```python
from build123d import *

# Parameters (mm, degrees)
SKETCH1_W           = 180
SKETCH1_H           = 77
SKETCH1_R           = 1.5
SKETCH1_R_2         = 1.500742376
BOSS_EXTRUDE1_DEPTH = 3
FILLET1_R           = 3
CUT_EXTRUDE1_DEPTH  = 3
SKETCH3_R           = 1.5
CUT_EXTRUDE2_DEPTH  = 3
SKETCH4_R           = 1.5
CUT_EXTRUDE3_DEPTH  = 3
SKETCH5_W           = 20
SKETCH5_H           = 34
BOSS_EXTRUDE2_DEPTH = 20
SKETCH6_R           = 1.5
CUT_EXTRUDE4_DEPTH  = 3


with BuildPart() as part:
    # Sketch1 → Boss-Extrude1 (new body)
    with BuildSketch(Plane(origin=(0, 0, 0), x_dir=(1, 0, 0), z_dir=(0, 1, 0))):
        Rectangle(SKETCH1_W, SKETCH1_H)
        with Locations(Location((-87, 35.25, 0), (0, 0, 270))):
            Circle(SKETCH1_R, mode=Mode.SUBTRACT)
        with Locations(Location((-87, -35.25, 0), (0, 0, 90))):
            Circle(SKETCH1_R, mode=Mode.SUBTRACT)
        with Locations(Location((-35.005408935, 34.5, 0), (0, 0, 270))):
            Circle(SKETCH1_R, mode=Mode.SUBTRACT)
        with Locations(Location((-35.005408935, -34.5, 0), (0, 0, 90))):
            Circle(SKETCH1_R, mode=Mode.SUBTRACT)
        with Locations(Location((74.494591065, 33.15, 0), (0, 0, 270))):
            Circle(SKETCH1_R_2, mode=Mode.SUBTRACT)
        with Locations(Location((74.494591065, -33.15, 0), (0, 0, 270))):
            Circle(SKETCH1_R, mode=Mode.SUBTRACT)
    extrude(amount=BOSS_EXTRUDE1_DEPTH)

    # Fillet1
    fillet1_edges = [part.edges().sort_by_distance(p)[0] for p in [
        (90, 1.5, 38.5),
        (-90, 1.5, 38.5),
        (-90, 1.5, -38.5),
        (90, 1.5, -38.5),
    ]]
    fillet(fillet1_edges, radius=FILLET1_R)

    # Sketch2 → Cut-Extrude1 (cut)
    with BuildSketch(Plane(origin=(0, 3, 0), x_dir=(1, 0, 0), z_dir=(0, 1, 0))):
        with BuildLine():
            Line((-62, 14.5), (-42, 14.5))
            ThreePointArc((-42, 14.5), (-41.292893219, 14.792893219), (-41, 15.5))
            Line((-41, 15.5), (-41, 28.5))
            ThreePointArc((-41, 28.5), (-41.292893219, 29.207106781), (-42, 29.5))
            Line((-42, 29.5), (-62, 29.5))
            ThreePointArc((-62, 29.5), (-62.707106781, 29.207106781), (-63, 28.5))
            Line((-63, 28.5), (-63, 15.5))
            ThreePointArc((-63, 15.5), (-62.707106781, 14.792893219), (-62, 14.5))
        make_face()
    extrude(amount=-CUT_EXTRUDE1_DEPTH, mode=Mode.SUBTRACT)

    # Sketch3 → Cut-Extrude2 (cut)
    with BuildSketch(Plane(origin=(0, 3, 0), x_dir=(1, 0, 0), z_dir=(0, 1, 0))):
        with Locations(Location((-79.5, 3.75, 0), (0, 0, 270))):
            Circle(SKETCH3_R)
        with Locations(Location((-42.5, 3.75, 0), (0, 0, 270))):
            Circle(SKETCH3_R)
        with Locations(Location((-42.5, -33.25, 0), (0, 0, 270))):
            Circle(SKETCH3_R)
        with Locations(Location((-79.5, -33.25, 0), (0, 0, 270))):
            Circle(SKETCH3_R)
    extrude(amount=-CUT_EXTRUDE2_DEPTH, mode=Mode.SUBTRACT)

    # Sketch4 → Cut-Extrude3 (cut)
    with BuildSketch(Plane(origin=(0, 3, 0), x_dir=(1, 0, 0), z_dir=(0, 1, 0))):
        with Locations(Location((-30.005408935, 24.25, 0), (0, 0, 270))):
            Circle(SKETCH4_R)
        with Locations(Location((52.994591065, 24.25, 0), (0, 0, 270))):
            Circle(SKETCH4_R)
        with Locations(Location((51.994591065, -24.25, 0), (0, 0, 270))):
            Circle(SKETCH4_R)
        with Locations(Location((-23.005408935, -24.25, 0), (0, 0, 270))):
            Circle(SKETCH4_R)
    extrude(amount=-CUT_EXTRUDE3_DEPTH, mode=Mode.SUBTRACT)

    # Sketch5 → Boss-Extrude2 (add)
    with BuildSketch(Plane.XZ):
        with Locations((40, 1.5)):
            Rectangle(SKETCH5_W, SKETCH5_H)
    extrude(amount=BOSS_EXTRUDE2_DEPTH)

    # Sketch6 → Cut-Extrude4 (cut)
    with BuildSketch(Plane.XZ):
        with Locations(Location((-14.5, -35.25, 0), (0, 0, 270))):
            Circle(SKETCH6_R)
        with Locations(Location((4.5, -35.25, 0), (0, 0, 270))):
            Circle(SKETCH6_R)
        with Locations(Location((4.5, 35.25, 0), (0, 0, 270))):
            Circle(SKETCH6_R)
        with Locations(Location((-14.5, 35.25, 0), (0, 0, 270))):
            Circle(SKETCH6_R)
        with Locations(Location((-5, -30.25, 0), (0, 0, 270))):
            Circle(SKETCH6_R)
        with Locations(Location((-5, 30.25, 0), (0, 0, 270))):
            Circle(SKETCH6_R)
    extrude(amount=-CUT_EXTRUDE4_DEPTH, mode=Mode.SUBTRACT)


solid = part.part
```
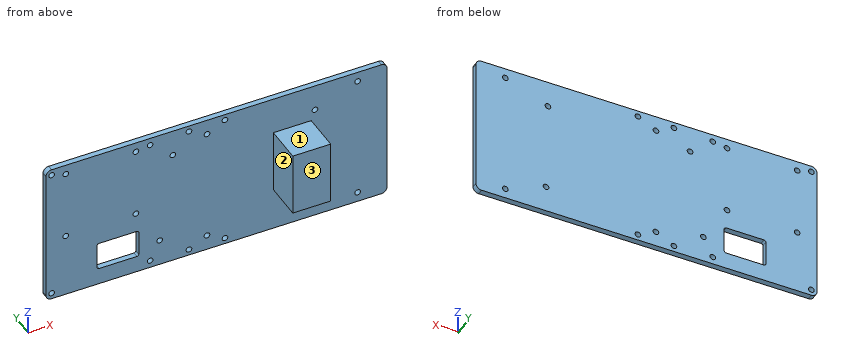
Geometry: final body of the model. Coordinates: model frame, mm. Face numbers are marked on the shaded views. A direction names the side the tool comes from. Give positions to 0.01 mm unless a question says otherwise; leave off trailing zeros. Loops run counter-clockwise (first coordinate to the right, second up) from the corner with the lowest first, then second, coordinate; pieces in that order, holes last. Notation, with made-up numbers: (37, -6) -> (45, -6) arc R7 cw to (45, -1) -> close; hole circle Ø3 at (11.5, -19). An arc over 180 degrees is marked (long way). Use CSV: the item, a comma, the result in double quotes.
(1) First-contact query: P1, Ø3, axis at x = 1, z = -5.5, coming from the -Y side. Flat tip, straight axial feed; report the tip coordinate or a pass-through.
From the geometry:
P1,"y = 0"
(2) Cut plane C-C (x = -66). Output: boundary loops of the cut face in (y, z), plus the area to 3 significant figures.
From the geometry:
outline,"(0, -38.5) -> (3, -38.5) -> (3, 38.5) -> (0, 38.5) -> close"
area,"231 mm^2"
(3) Access query for the marked faces 1, 2 and 3. Directions: +Z, -Z, +X, -X, +Y, -Y. A direction counts if a zero-diameter tool reaches every point of the face in a straight line with its end or side. Return the directions, or none.
From the geometry:
face 1,"+Z, +X, -X, -Y"
face 2,"+Z, -Z, -X, -Y"
face 3,"+Z, -Z, +X, -X, -Y"
(4) Ray query, line 1 along X through (y, z) = (2.4, -3.75); line 2 along X through (y, z) = (2, -24.25); line 3 along Z through (x, y) = (-87, 1). Return the intervals inside material, ascending. Write a range as [from, to].
From the geometry:
line 1,"[-90, -81], [-78, -44], [-41, 90]"
line 2,"[-90, -63], [-41, -31.51], [-28.51, 51.49], [54.49, 90]"
line 3,"[-38.5, -36.75], [-33.75, 33.75], [36.75, 38.5]"
(5) Cut plane B-B (y = -14.25). Output: boundary loops of the cut face in (x, z), plus the area to 3 significant figures.
From the geometry:
outline,"(30, -15.5) -> (50, -15.5) -> (50, 18.5) -> (30, 18.5) -> close"
area,"680 mm^2"
(6) Cut plane A-A (z = 10). Output: boundary loops of the cut face in (x, y), plus the area to 3 significant figures.
From the geometry:
outline,"(-90, 0) -> (30, 0) -> (30, -20) -> (50, -20) -> (50, 0) -> (90, 0) -> (90, 3) -> (-90, 3) -> close"
area,"940 mm^2"
